from build123d import *

# Parameters (mm, degrees)
SKETCH1_R           = 40
BOSS_EXTRUDE1_DEPTH = 714
CHAMFER1_SIZE       = 3


with BuildPart() as part:
    # Sketch1 → Boss-Extrude1 (new, symmetric)
    with BuildSketch(Plane.XY):
        Circle(SKETCH1_R)
    extrude(amount=BOSS_EXTRUDE1_DEPTH, both=True)

    # Sketch2 → Cut-Revolve1 (revolve, cut)
    with BuildSketch(Plane(origin=(0, 0, 0), x_dir=(0, 0, -1), z_dir=(1, 0, 0)), mode=Mode.PRIVATE) as cut_revolve1_sk:
        Polygon((-714, 34), (-654, 34), (-654, 35), (-634, 35), (-634, 52.852263241), (-714, 52.852263241), align=None)
    revolve(cut_revolve1_sk.sketch.rotate(Axis((0, 0, 0), (0, 0, 1)), 90), axis=Axis((0, 0, 0), (0, 0, 1)), mode=Mode.SUBTRACT)

    # Chamfer1
    # the kernel refuses this chamfer: 3 mm, written as the material it takes off along each edge
    with BuildSketch(Plane(origin=(0, 0, 654), x_dir=(-1, 0, 0), z_dir=(0, 1, 0))) as chamfer1_piece_1_section:
        Polygon((35, -CHAMFER1_SIZE), (35 - CHAMFER1_SIZE, 0), (35, 0), align=None)
    chamfer1_piece_1 = revolve(axis=Axis((0, 0, 654), (0, 0, 1)), mode=Mode.PRIVATE)
    chamfer1_piece_1 = chamfer1_piece_1 - Plane(origin=(0, 0, 651.51733658), x_dir=(-1, 0, 0), z_dir=(0, 0, -1)) * Cylinder(34, 140, mode=Mode.PRIVATE)
    add(chamfer1_piece_1, mode=Mode.SUBTRACT)
    with BuildSketch(Plane(origin=(0, 0, 714), x_dir=(-1, 0, 0), z_dir=(0, 1, 0))) as chamfer1_piece_2:
        Polygon((34, -CHAMFER1_SIZE), (34 - CHAMFER1_SIZE, 0), (34, 0), align=None)
    revolve(axis=Axis((0, 0, 714), (0, 0, 1)), mode=Mode.SUBTRACT)


solid = part.part
Could you check a few things on this model? Use its own coordinates, in mm. A direction names the side the tool comes from. Coordinates: 2 decimals unless noted, no trailing zeros. Loops run counter-clockwise (first coordinate to the right, second up) from the corner with the lowest first, then second, coordinate; pieces in that order, holes last.
1. For P1, Ø10, axis at x = 9, z = -115, coming from the -Y side; P2, Ø8, axis at y = 31.5, z = -389, coming from the +X side; P3, Ø1, axis at y = -5.5, z = -522.5, coming from the +X side, each with a flat end and sliding along its axis, tell me the tip position at first contact or that it passes through.
2. I need wall thicknesses on L1, parallel to Z at x = -30, y = -19.5; L2, parallel to Y at x = -2.5, z = 380.5; L3, parallel to X at y = 21.5, z = -189.5. Which ranges of each line are inside material? Lowest first, please.
3. Imagine slicing it at A-A (z = 468). Please give me the cut outline in (x, y), and give its area (3 significant figures).
4. For faces 1 (the face through (-0.2, 35.4, 634)), 2 (the face through (0, 0, 714)), which set-ups out of +Z, -Z, +X, -X, +Y, -Y let a thin tool reach every point of the face, with its end or its side?
Computed values:
1. P1: stops at y = -39.8
1. P2: stops at x = 29.05
1. P3: stops at x = 39.69
2. L1: z = -714 to 634
2. L2: y = -39.92 to 39.92
2. L3: x = -33.73 to 33.73
3. outline: circle Ø80 at (0, 0)
3. area: 5,030 mm2
4. face 1: +Z
4. face 2: +Z, +X, -X, +Y, -Y
